Geometry check sheet. Reference: the model listing, model coordinates, mm. A direction names the side the tool comes from. Coordinates: 2 decimals unless noted, no trailing zeros. Write each question's results on one line, items separated by ' | '.
```python
from build123d import *

# Parameters (mm, degrees)
BOSS_EXTRUDE1_DEPTH     = 76.2
CUT_EXTRUDE1_DEPTH      = 77.2
CUT_EXTRUDE1_DEPTH_BACK = 77.2


with BuildPart() as part:
    # Sketch4 → Boss-Extrude1 (new body, symmetric)
    with BuildSketch(Plane.XY):
        with BuildLine():
            Line((20, -17), (20, -5.32))
            ThreePointArc((20, -5.32), (19.613380951, -4.386619049), (18.68, -4))
            Line((18.68, -4), (18.02, -4))
            ThreePointArc((18.02, -4), (17.086619049, -4.386619049), (16.7, -5.32))
            Line((16.7, -5.32), (16.7, -6.75))
            Line((16.7, -6.75), (17.36, -6.75))
            Line((17.36, -6.75), (17.36, -10.4))
            ThreePointArc((17.36, -10.4), (17.184264069, -10.824264069), (16.76, -11))
            Line((16.76, -11), (13.11529004, -11))
            ThreePointArc((13.11529004, -11), (12.88567998, -10.95432772), (12.691025971, -10.824264069))
            Line((12.691025971, -10.824264069), (8.386619049, -6.519857147))
            ThreePointArc((8.386619049, -6.519857147), (8.100479017, -6.091618326), (8, -5.586476195))
            Line((8, -5.586476195), (8, 0))
            Line((8, 0), (3.5, 0))
            ThreePointArc((3.5, 0), (2.474873734, -2.474873734), (0, -3.5))
            Line((0, -3.5), (0, -8))
            Line((0, -8), (5.586476195, -8))
            ThreePointArc((5.586476195, -8), (6.091618326, -8.100479017), (6.519857147, -8.386619049))
            Line((6.519857147, -8.386619049), (10.824264069, -12.691025971))
            ThreePointArc((10.824264069, -12.691025971), (10.95432772, -12.88567998), (11, -13.11529004))
            Line((11, -13.11529004), (11, -16.76))
            ThreePointArc((11, -16.76), (10.824264069, -17.184264069), (10.4, -17.36))
            Line((10.4, -17.36), (6.75, -17.36))
            Line((6.75, -17.36), (6.75, -16.7))
            Line((6.75, -16.7), (5.32, -16.7))
            ThreePointArc((5.32, -16.7), (4.386619049, -17.086619049), (4, -18.02))
            Line((4, -18.02), (4, -18.68))
            ThreePointArc((4, -18.68), (4.386619049, -19.613380951), (5.32, -20))
            Line((5.32, -20), (17, -20))
            ThreePointArc((17, -20), (19.121320344, -19.121320344), (20, -17))
        make_face()
        with BuildLine():
            Line((15.68, -18.68), (12.32, -18.68))
            Line((12.32, -18.68), (12.32, -12.32))
            Line((12.32, -12.32), (18.68, -12.32))
            Line((18.68, -12.32), (18.68, -15.68))
            ThreePointArc((18.68, -15.68), (17.801320344, -17.801320344), (15.68, -18.68))
        make_face(mode=Mode.SUBTRACT)
    extrude(amount=BOSS_EXTRUDE1_DEPTH, both=True)

    # Mirror1: part across plane


with BuildPart() as part_1:
    add(part.part)
    add(part.part.mirror(Plane(origin=(0, 0, 0), x_dir=(0, 0, 1), z_dir=(1, 0, 0))))

    # Mirror2: part across plane


with BuildPart() as part_2:
    add(part_1.part)
    add(part_1.part.mirror(Plane.ZX))

    # Sketch5 → Cut-Extrude1 (cut, two sides)
    with BuildSketch(Plane.XY) as cut_extrude1_sk:
        Polygon((-10.453238098, 12.32), (-10.453238098, 11.99), (-10.123238098, 11.99), (-9.88989286, 11.756654762), (-9.88989286, 11.426654762), (-9.55989286, 11.426654762), (-9.55989286, 12.32), align=None)
    extrude(amount=CUT_EXTRUDE1_DEPTH, mode=Mode.SUBTRACT)
    extrude(cut_extrude1_sk.sketch, amount=-CUT_EXTRUDE1_DEPTH_BACK, mode=Mode.SUBTRACT)


solid = part_2.part
```
Q1. Access from +Z, -Z, +X, -X, +Y, -Y to the whole of each face (thin tool, end or side, straight path). Record for faces 1 (the flat face through (20, 11, 1)), 2 (the flat face through (15, 12.32, 1)).
Geometry check:
face 1: +Z, -Z, +X, +Y, -Y | face 2: +Z, -Z
Q2. Depth check by flat-ended pin: P1, Ø4, axis at y = -1, z = 51, coming from the +X side; P2, Ø0.5, axis at y = -18.5, z = 24, coming from the -X side; P3, Ø1, axis at x = 0, z = -48.5, coming from the -Y side. Enter the tip coordinate at first touch or a pass-through.
Geometry check:
P1: stops at x = 8 | P2: stops at x = -19.73 | P3: stops at y = -8
Q3. Scan lines: probe 1 along Y at (x, z) = (15, 31); probe 2 along X at (y, z) = (5.5, 26). Record each from-to range of solid material in increasing order.
Geometry check:
probe 1: y = -20 to -18.68, -12.32 to -11, 11 to 12.32, 18.68 to 20 | probe 2: x = -20 to -16.7, -8 to 8, 16.7 to 20
Q4. Sectioned sample at A-A on z = 26.5. Give the number of separate pieces and of enclosed holes in the cut face, and give its area (3 significant figures).
Geometry check:
separate pieces: 1 | enclosed holes: 5 | area: 596 mm2
Q5. Mould release check, pull along Y, two halves, no side actions. Record for faces 3 (the flat face through (11, -20, 1)), 4 (the flat face through (-11, 20, 1)), 5 (the flat face through (17.36, -9, 1)): pulls with the +Y half, pulls with the -Y half, needs draft (parallel to the pull), parting line crosses it, or undercut.
Geometry check:
face 3: pulls with the -Y half | face 4: pulls with the +Y half | face 5: undercut
